from build123d import *

# Parameters (mm, degrees)
F0_R     = 2.15
F1_DEPTH = 50


with BuildPart() as f1:
    # F0 (on Top) → F1 (new body)
    with BuildSketch(Plane.XY):
        with BuildLine():
            Line((-2.699069, 10), (-9.7, 10))
            ThreePointArc((-9.7, 10), (-9.912132, 9.912132), (-10, 9.7))
            Line((-10, 9.7), (-10, 2.699069))
            ThreePointArc((-10, 2.699069), (-9.941694, 2.558306), (-9.800931, 2.5))
            Line((-9.800931, 2.5), (-8.449069, 2.5))
            ThreePointArc((-8.449069, 2.5), (-8.308306, 2.558306), (-8.25, 2.699069))
            Line((-8.25, 2.699069), (-8.25, 4.730027))
            ThreePointArc((-8.25, 4.730027), (-8.153763, 4.90048), (-7.958101, 4.906127))
            Line((-7.958101, 4.906127), (-4.183679, 2.916455))
            ThreePointArc((-4.183679, 2.916455), (-3.793752, 2.548405), (-3.65, 2.03184))
            Line((-3.65, 2.03184), (-3.65, 0))
            Line((-3.65, 0), (-3.65, -2.03184))
            ThreePointArc((-3.65, -2.03184), (-3.793752, -2.548405), (-4.183679, -2.916455))
            Line((-4.183679, -2.916455), (-7.958101, -4.906127))
            ThreePointArc((-7.958101, -4.906127), (-8.153763, -4.90048), (-8.25, -4.730027))
            Line((-8.25, -4.730027), (-8.25, -2.699069))
            ThreePointArc((-8.25, -2.699069), (-8.308306, -2.558306), (-8.449069, -2.5))
            Line((-8.449069, -2.5), (-9.800931, -2.5))
            ThreePointArc((-9.800931, -2.5), (-9.941694, -2.558306), (-10, -2.699069))
            Line((-10, -2.699069), (-10, -9.7))
            ThreePointArc((-10, -9.7), (-9.912132, -9.912132), (-9.7, -10))
            Line((-9.7, -10), (-2.699069, -10))
            ThreePointArc((-2.699069, -10), (-2.558306, -9.941694), (-2.5, -9.800931))
            Line((-2.5, -9.800931), (-2.5, -8.449069))
            ThreePointArc((-2.5, -8.449069), (-2.558306, -8.308306), (-2.699069, -8.25))
            Line((-2.699069, -8.25), (-4.730027, -8.25))
            ThreePointArc((-4.730027, -8.25), (-4.90048, -8.153763), (-4.906127, -7.958101))
            Line((-4.906127, -7.958101), (-2.916455, -4.183679))
            ThreePointArc((-2.916455, -4.183679), (-2.548405, -3.793752), (-2.03184, -3.65))
            Line((-2.03184, -3.65), (0, -3.65))
            Line((0, -3.65), (2.03184, -3.65))
            ThreePointArc((2.03184, -3.65), (2.548405, -3.793752), (2.916455, -4.183679))
            Line((2.916455, -4.183679), (4.906127, -7.958101))
            ThreePointArc((4.906127, -7.958101), (4.90048, -8.153763), (4.730027, -8.25))
            Line((4.730027, -8.25), (2.699069, -8.25))
            ThreePointArc((2.699069, -8.25), (2.558306, -8.308306), (2.5, -8.449069))
            Line((2.5, -8.449069), (2.5, -9.800931))
            ThreePointArc((2.5, -9.800931), (2.558306, -9.941694), (2.699069, -10))
            Line((2.699069, -10), (9.7, -10))
            ThreePointArc((9.7, -10), (9.912132, -9.912132), (10, -9.7))
            Line((10, -9.7), (10, -2.699069))
            ThreePointArc((10, -2.699069), (9.941694, -2.558306), (9.800931, -2.5))
            Line((9.800931, -2.5), (8.449069, -2.5))
            ThreePointArc((8.449069, -2.5), (8.308306, -2.558306), (8.25, -2.699069))
            Line((8.25, -2.699069), (8.25, -4.730027))
            ThreePointArc((8.25, -4.730027), (8.153763, -4.90048), (7.958101, -4.906127))
            Line((7.958101, -4.906127), (4.183679, -2.916455))
            ThreePointArc((4.183679, -2.916455), (3.793752, -2.548405), (3.65, -2.03184))
            Line((3.65, -2.03184), (3.65, 0))
            Line((3.65, 0), (3.65, 2.03184))
            ThreePointArc((3.65, 2.03184), (3.793752, 2.548405), (4.183679, 2.916455))
            Line((4.183679, 2.916455), (7.958101, 4.906127))
            ThreePointArc((7.958101, 4.906127), (8.153763, 4.90048), (8.25, 4.730027))
            Line((8.25, 4.730027), (8.25, 2.699069))
            ThreePointArc((8.25, 2.699069), (8.308306, 2.558306), (8.449069, 2.5))
            Line((8.449069, 2.5), (9.800931, 2.5))
            ThreePointArc((9.800931, 2.5), (9.941694, 2.558306), (10, 2.699069))
            Line((10, 2.699069), (10, 9.7))
            ThreePointArc((10, 9.7), (9.912132, 9.912132), (9.7, 10))
            Line((9.7, 10), (2.699069, 10))
            ThreePointArc((2.699069, 10), (2.558306, 9.941694), (2.5, 9.800931))
            Line((2.5, 9.800931), (2.5, 8.449069))
            ThreePointArc((2.5, 8.449069), (2.558306, 8.308306), (2.699069, 8.25))
            Line((2.699069, 8.25), (4.730027, 8.25))
            ThreePointArc((4.730027, 8.25), (4.90048, 8.153763), (4.906127, 7.958101))
            Line((4.906127, 7.958101), (2.916455, 4.183679))
            ThreePointArc((2.916455, 4.183679), (2.548405, 3.793752), (2.03184, 3.65))
            Line((2.03184, 3.65), (0, 3.65))
            Line((0, 3.65), (-2.03184, 3.65))
            ThreePointArc((-2.03184, 3.65), (-2.548405, 3.793752), (-2.916455, 4.183679))
            Line((-2.916455, 4.183679), (-4.906127, 7.958101))
            ThreePointArc((-4.906127, 7.958101), (-4.90048, 8.153763), (-4.730027, 8.25))
            Line((-4.730027, 8.25), (-2.699069, 8.25))
            ThreePointArc((-2.699069, 8.25), (-2.558306, 8.308306), (-2.5, 8.449069))
            Line((-2.5, 8.449069), (-2.5, 9.800931))
            ThreePointArc((-2.5, 9.800931), (-2.558306, 9.941694), (-2.699069, 10))
        make_face()
        Circle(F0_R, mode=Mode.SUBTRACT)
    extrude(amount=F1_DEPTH)


solid = f1.part
Work out the finished part from the listing and answer in its coordinate system (mm). A direction names the side the tool comes from. Round coordinates to 2 decimals unless told otherwise and drop trailing zeros. Order: outer loops, then holes, each group sorted by start corner. A loop starts at its lowest first (then second) coordinate and runs counter-clockwise, first axis right, second up. Notation, with made-up numbers: M 34.5,8 L 76.5,8 A18 ccw 76.5,12 Z; hole C -29,2 d5. An arc over 180 degrees is marked long. Put each result on its own line as item: value. Start each with the question number.
Q1. For a pull along Y with two mould halves and no side action, classify faces 5 (the flat face through (6, 10, 25)), 6 (the flat face through (10, 6, 25)), 7 (the flat face through (4, -8.25, 25)) as pulls with the +Y half, pulls with the -Y half, needs draft (parallel to the pull), parting line crosses it, or undercut.
Q2. Straight lines are drawn through the part: L1, parallel to X at y = -8, z = 29; L2, parallel to X at y = -3.5, z = 21.5; L3, parallel to Y at x = 0, z = 29.5. For each, find the intervals that lie inside material, in ascending order. Write a range as [from, to].
Q3. Section A-A, the plane y = 0 is taken. Write down the section's boundary in (x, z), and give its area (3 significant figures).
Q4. A tool of negligible diameter and unlimited length cuts with its end or side. For faces 1 (the flat face through (9, 2.5, 25)), 2 (the flat face through (-2.5, 9, 25)), 3 (the flat face through (-9, 2.5, 25)), 4 (the flat face through (-4, -8.25, 25)), from which of +Z, -Z, +X, -X, +Y, -Y can it reach the whole face along a straight path? Write none if from no direction.
Q5. Flat-ended cylindrical pins translate along their axes: pin 1 (1.5 mm diameter, centred on x = 6, y = 1.5, fed in from -Z); pin 2 (1.2 mm diameter, centred on x = 0.5, z = 27, fed in from +Y). Find the tip coordinate at first contact, or state that the pin passes through.
Findings below:
1. face 5: pulls with the +Y half
1. face 6: needs draft
1. face 7: undercut
2. L1: x = [-10, -4.92], [4.92, 10]
2. L2: x = [-10, -8.25], [-5.29, 5.29], [8.25, 10]
2. L3: y = [-3.65, -2.15], [2.15, 3.65]
3. outline: M -3.65,0 L -2.15,0 L -2.15,50 L -3.65,50 Z; M 2.15,0 L 3.65,0 L 3.65,50 L 2.15,50 Z
3. area: 150 mm^2
4. face 1: +Z, -Z, +X
4. face 2: +Z, -Z, +Y
4. face 3: +Z, -Z, -X
4. face 4: +Z, -Z
5. pin 1: passes through
5. pin 2: stops at y = 3.65
